Could you check a few things on this drawing? It's one solid part, dimensions in mm from its lowest x, y, z. Coordinates: 2 decimals unless noted, no trailing zeros. Order: outer loops, then holes, each group sorted by start corner. A loop starts at its lowest first (then second) coordinate and runs counter-clockwise, first axis right, second up. Notation, with made-up numbers: (23.25, -3) -> (41.25, -3) arc R13 cw to (41.25, 18) -> close; hole circle Ø3 at (-35.75, 63.5). An arc over 180 degrees is marked (long way). Use a Markdown table: item, result. Add a question column.
1. Suppose I cut it at A-A, the plane y = 2.5. List the corners of the cut face in (x, z) for me (1 decimal), then the cut area to 3 significant figures.
2. If I drill on line 1 along Z through (x, y) = (213, 7.25) (1 decimal); line 2 along Z through (x, y) = (32, 7.5), over which ranges is the centre line in solid material (lowest first)? Write a range as from..to.
3. Suppose I cut it at B-B, the plane z = 27. List the corners of the cut face in (x, y) for me.
4. Suppose I cut it at C-C, the plane x = 154. List the corners of the cut face in (y, z) for me.
5. For pin 1 Ø1.5 at (x, y) = (116.5, 1.5) entering from -Z (1 decimal); pin 2 Ø1.5 at (y, z) = (13, 91.5) entering from -X, each with a flat end and sliding along its axis, tell me the tip position at first contact or that it passes through.
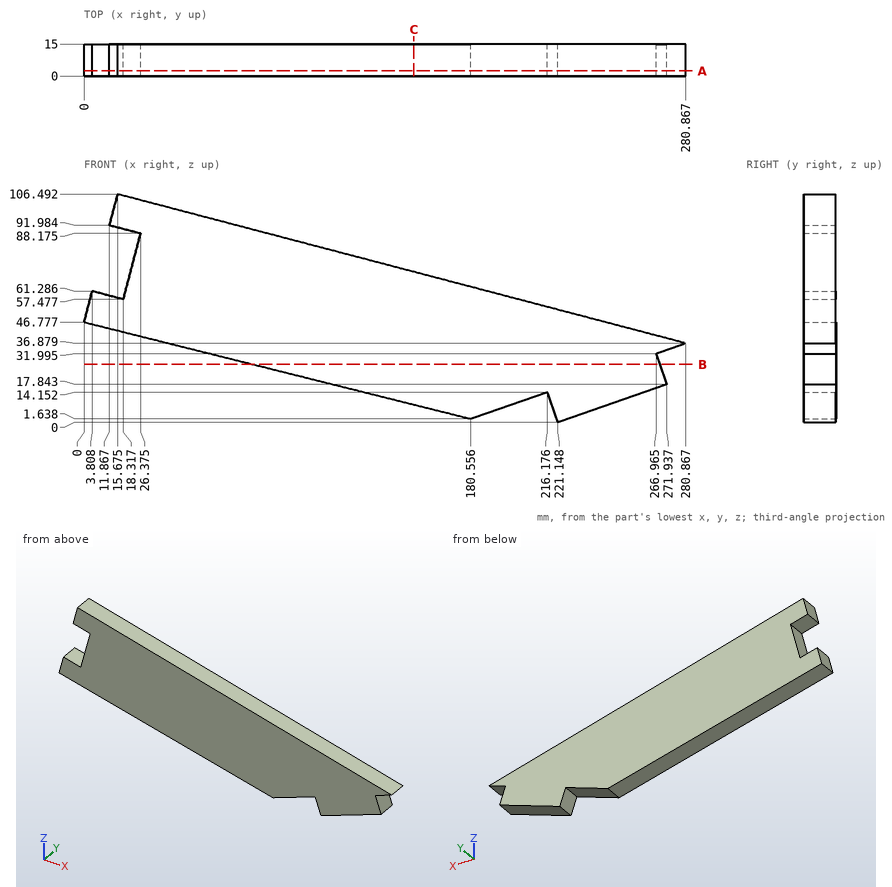
Worked out:
| question | item | result |
|---|---|---|
| 1 | outline | (0, 46.8) -> (180.6, 1.6) -> (216.2, 14.2) -> (221.1, 0) -> (271.9, 17.8) -> (267, 32) -> (280.9, 36.9) -> (15.7, 106.5) -> (11.9, 92) -> (26.4, 88.2) -> (18.3, 57.5) -> (3.8, 61.3) -> close |
| 1 | area | 14,200 mm² |
| 2 | line 1 | z = 13..54.7 |
| 2 | line 2 | z = 38.78..102.21 |
| 3 | outline | (79.11, 0) -> (268.72, 0) -> (268.72, 15) -> (79.11, 15) -> close |
| 4 | outline | (0, 8.28) -> (15, 8.28) -> (15, 70.18) -> (0, 70.18) -> close |
| 5 | pin 1 | stops at z = 17.5 |
| 5 | pin 2 | stops at x = 11.87 |
